Model file for the job. Use its own axes, mm. Face numbers are marked on the shaded views. A direction names the side the tool comes from. Coordinates: 2 decimals unless noted, no trailing zeros. Order: outer loops, then holes, each group sorted by start corner. A loop starts at its lowest first (then second) coordinate and runs counter-clockwise, first axis right, second up.
from build123d import *

# Parameters (mm, degrees)
F0_W     = 118.3868944645
F0_H     = 82.3358744383
F1_DEPTH = 68.326
F2_W     = 118.3868944645
F2_H     = 54.3707673127
F3_DEPTH = 55.88
F5_DEPTH = 25.4
F7_DEPTH = 87.122
F8_R     = 7.0278301123
F9_DEPTH = 25.4


with BuildPart() as f1:
    # F0 (on Front) → F1 (new body)
    with BuildSketch(Plane.XZ):
        with Locations((1.5118196607, 2.325873822)):
            Rectangle(F0_W, F0_H)
    extrude(amount=F1_DEPTH)

    # F2 (on face) → F3 (cut)
    with BuildSketch(Plane(origin=(0, 0, -38.8420633972), x_dir=(1, 0, 0), z_dir=(0, 0, -1))):
        with Locations((1.5118196607, 41.1406163436)):
            Rectangle(F2_W, F2_H)
    extrude(amount=-F3_DEPTH, mode=Mode.SUBTRACT)

    # F4 (on face) → F5 (cut)
    with BuildSketch(Plane.XZ.offset(13.9552326873)):
        Polygon((60.7052668929, -19.5373259485), (35.5858430266, -38.8420633972), (60.7052668929, -38.8420633972), align=None)
        Polygon((-57.6816275716, -38.8420633972), (-33.5003801701, -38.8420633972), (-57.6816275716, -18.3743909001), align=None)
    extrude(amount=-F5_DEPTH, mode=Mode.SUBTRACT)

    # F6 (on face) → F7 (cut)
    with BuildSketch(Plane.XZ.offset(68.326)):
        Polygon((40.9353487194, 28.1430520117), (32.7947959304, 43.4938110411), (-29.0733985603, 43.4938110411), (-37.2139513493, 28.1430520117), align=None)
    extrude(amount=-F7_DEPTH, mode=Mode.SUBTRACT)

    # F8 (on face) → F9 (cut)
    with BuildSketch(Plane(origin=(0, 0, 17.0379366028), x_dir=(1, 0, 0), z_dir=(0, 0, -1))):
        with Locations((0, 42.8269580007)):
            Circle(F8_R)
    extrude(amount=-F9_DEPTH, mode=Mode.SUBTRACT)


solid = f1.part
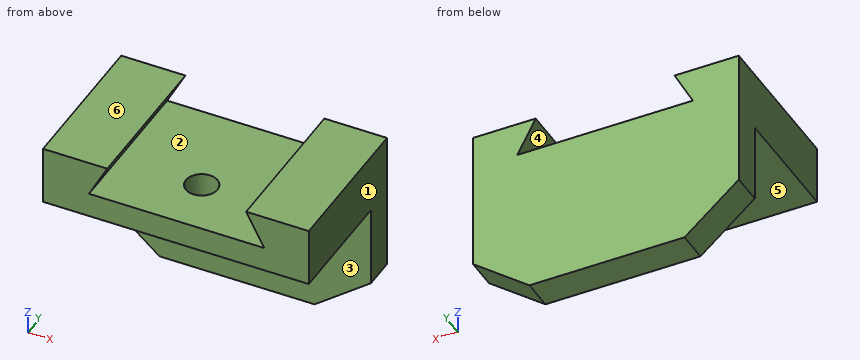
Q1. Drop flat-ended pins along their axis: P1, Ø1, axis at x = -19, z = -28.5, coming from the -Y side; P2, Ø6, axis at x = 25.5, y = -58.5, coming from the +Z side; P3, Ø6, axis at x = 46, y = -37.5, coming from the -Z side. Give the stop position or say it passes through.
Established:
P1: stops at y = -13.96
P2: stops at z = 28.14
P3: stops at z = 17.04
Q2. Cut at B-B, the plane y = -55. List the corners of the cut face in (x, z), plus the area to 3 significant figures.
Established:
outline: (-57.68, 17.04) - (60.71, 17.04) - (60.71, 43.49) - (32.79, 43.49) - (40.94, 28.14) - (-37.21, 28.14) - (-29.07, 43.49) - (-57.68, 43.49) - close
area: 2,060 mm2
Q3. Cut at D-D, the plane z = 33.5. List the corners of the cut face in (x, y).
Established:
outline: (-57.68, -68.33) - (-34.37, -68.33) - (-34.37, 0) - (-57.68, 0) - close; (38.09, -68.33) - (60.71, -68.33) - (60.71, 0) - (38.09, 0) - close
Q4. Cut at C-C, the plane x = -21. List the corners of the cut face in (y, z), plus the area to 3 significant figures.
Established:
outline: (-68.33, 17.04) - (-13.96, 17.04) - (-13.96, -38.84) - (0, -38.84) - (0, 28.14) - (-68.33, 28.14) - close
area: 1,540 mm2
Q5. Probe line 1 (Y direction, x = 0, z = 23); line 2 (Z direction, x = 20, y = -19); line 3 (Y direction, x = 49.5, z = -16.5). List the from-to ranges inside material, lowest first.
Established:
line 1: y = -68.33 to -49.85, -35.8 to 0
line 2: z = 17.04 to 28.14
line 3: y = -13.96 to 0
Q6. Cut at A-A, the plane x = 0. List the corners of the cut face in (y, z), plus the area to 3 significant figures.
Established:
outline: (-68.33, 17.04) - (-49.85, 17.04) - (-49.85, 28.14) - (-68.33, 28.14) - close; (-35.8, 17.04) - (-13.96, 17.04) - (-13.96, -38.84) - (0, -38.84) - (0, 28.14) - (-35.8, 28.14) - close
area: 1,380 mm2
Q7. Mould opens along X. For the marked faces 1, 2 and 3 say: pulls with the +X half, pulls with the -X half, needs draft (parallel to the pull), parting line crosses it, or undercut.
Established:
face 1: pulls with the +X half
face 2: undercut
face 3: needs draft
Q8. Which spindle directions (+Z, -Z, +X, -X, +Y, -Y) get a long thin tool onto all of the face, cutting with end or side? Do the marked faces 4, 5 and 6. Say none if no direction does.
Established:
face 4: +Y, -Y
face 5: -Z, +X, -X, -Y
face 6: +Z, +X, -X, +Y, -Y
